Can you work these out from the drawing? Everything is in mm from the part's minimum corner. Coordinates: 2 decimals unless noted, no trailing zeros. Order: outer loops, then holes, each group sorted by start corner. A loop starts at its lowest first (then second) coordinate and runs counter-clockwise, first axis right, second up. Notation, with made-up numbers: (72.5, 67.25) - (93.5, 67.25) arc R27 ccw to (93.5, 94.25) - close; hole circle Ø6 at (-4.75, -15.5). An arc over 180 degrees is marked (long way). One line per item, written item: value.
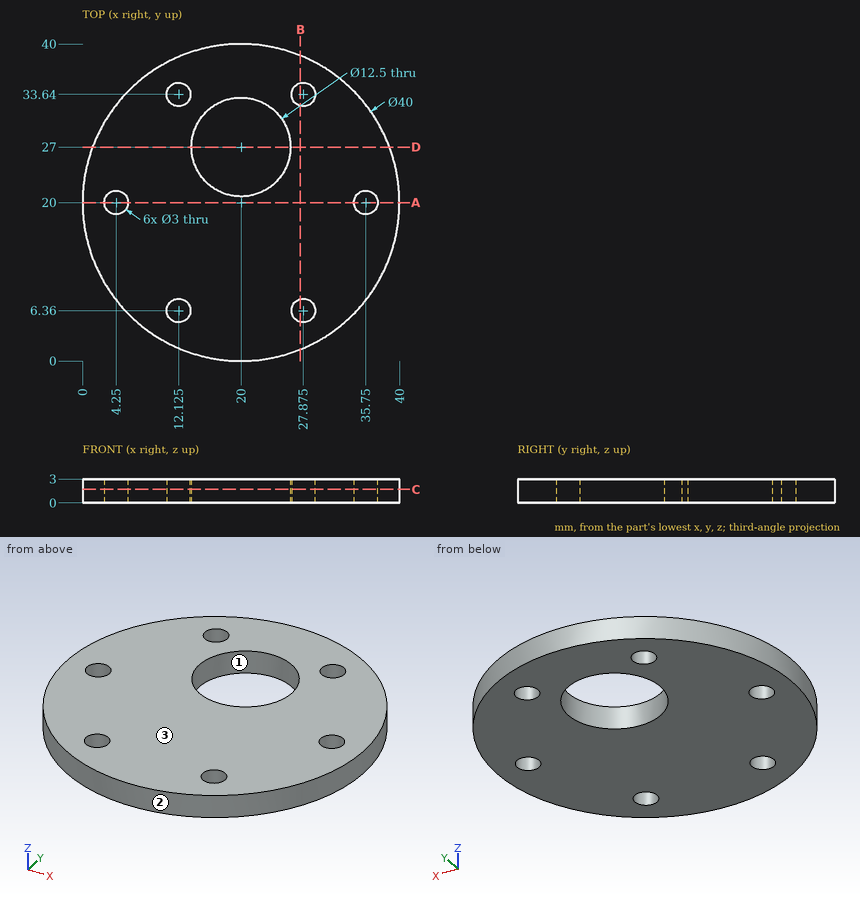
Item 1: I'm going to push flat-ended pins straight in: pin 1 Ø10 at (x, y) = (20, 27) entering from +Z; pin 2 Ø1 at (x, z) = (5, 2.5) entering from -Y (3 decimals). Where does each tip first touch, or does it pass through?
Conclusion:
pin 1: through
pin 2: y = 6.225
Item 2: I want a section at B-B on x = 27.5. Please give me the cut outline in (y, z).
Conclusion:
outline: (1.46, 0) - (4.91, 0) - (4.91, 3) - (1.46, 3) - close; (7.81, 0) - (32.19, 0) - (32.19, 3) - (7.81, 3) - close; (35.09, 0) - (38.54, 0) - (38.54, 3) - (35.09, 3) - close
Item 3: If I drill on probe 1 along X at (y, z) = (35, 0.3); probe 2 along X at (y, z) = (25.5, 1.85); probe 3 along Y at (x, z) = (21, 2.75) (1 decimal), over which ranges is the centre line in solid material (lowest first)?
Conclusion:
probe 1: 6.77 to 11.49, 12.76 to 27.24, 28.51 to 33.23
probe 2: 0.77 to 13.93, 26.07 to 39.23
probe 3: 0 to 20.8, 33.2 to 40
Item 4: I want a section at C-C on z = 1.7. Please give me the cut outline in (x, y) (3 decimals).
Conclusion:
outline: circle Ø40 at (20, 20); hole circle Ø3 at (4.25, 20); hole circle Ø3 at (12.125, 6.36); hole circle Ø3 at (12.125, 33.64); hole circle Ø12.5 at (20, 27); hole circle Ø3 at (27.875, 6.36); hole circle Ø3 at (27.875, 33.64); hole circle Ø3 at (35.75, 20)
Item 5: Thinking about a two-plate mould opening in Y: for the marked faces 1, 2 and 3, which applies, pulls with the +Y half, pulls with the -Y half, needs draft (parallel to the pull), parting line crosses it, or undercut?
Conclusion:
face 1: undercut
face 2: parting line crosses it
face 3: needs draft
Item 6: I want a section at D-D on y = 27. Please give me the cut outline in (x, z) (3 decimals), then the cut area to 3 significant figures.
Conclusion:
outline: (1.265, 0) - (13.75, 0) - (13.75, 3) - (1.265, 3) - close; (26.25, 0) - (38.735, 0) - (38.735, 3) - (26.25, 3) - close
area: 74.9 mm²
Item 7: I want a section at A-A on y = 20. Please give me the cut outline in (x, z), then the cut area to 3 significant figures.
Conclusion:
outline: (0, 0) - (2.75, 0) - (2.75, 3) - (0, 3) - close; (5.75, 0) - (34.25, 0) - (34.25, 3) - (5.75, 3) - close; (37.25, 0) - (40, 0) - (40, 3) - (37.25, 3) - close
area: 102 mm²
